```python
from build123d import *

# Parameters (mm, degrees)
SKETCH1_R                 = 25
BOSS_EXTRUDE1_DEPTH       = 10
FILLET1_R                 = 1
SKETCH2_R                 = 8
BOSS_EXTRUDE2_DEPTH       = 63.5
M8X1_0_TAPPED_HOLE1_D     = 7
M8X1_0_TAPPED_HOLE1_DEPTH = 12
M8X1_0_TAPPED_HOLE1_TIP   = 2.103012167
SKETCH5_OUTSIDE_W         = 72.398
SKETCH5_OUTSIDE_H         = 72.398
SKETCH5_OUTSIDE_W_2       = 13
SKETCH5_OUTSIDE_H_2       = 18.1448046
CUT_EXTRUDE1_DEPTH        = 5


with BuildPart() as part:
    # Sketch1 → Boss-Extrude1 (new body)
    with BuildSketch(Plane(origin=(0, 0, 0), x_dir=(1, 0, 0), z_dir=(0, 1, 0))):
        with Locations(Location((0, 0, 0), (0, 0, 270))):
            Circle(SKETCH1_R)
    extrude(amount=BOSS_EXTRUDE1_DEPTH)

    # Fillet1
    fillet1_edges = [part.edges().sort_by_distance(p)[0] for p in [
        (0, 0, -25),
        (0, 10, -25),
    ]]
    fillet(fillet1_edges, radius=FILLET1_R)

    # Sketch2 → Boss-Extrude2 (add)
    with BuildSketch(Plane(origin=(0, 10, 0), x_dir=(1, 0, 0), z_dir=(0, 1, 0))):
        with Locations(Location((0, 0, 0), (0, 0, 270))):
            Circle(SKETCH2_R)
    extrude(amount=BOSS_EXTRUDE2_DEPTH)

    # M8x1.0 Tapped Hole1
    with Locations(Plane(origin=(0, 73.5, 0), x_dir=(1, 0, 0), z_dir=(0, 1, 0))):
        with Locations((0, 0)):
            Hole(M8X1_0_TAPPED_HOLE1_D / 2, depth=M8X1_0_TAPPED_HOLE1_DEPTH)
            with Locations((0, 0, -(M8X1_0_TAPPED_HOLE1_DEPTH + M8X1_0_TAPPED_HOLE1_TIP / 2))):  # 118° drill point
                Cone(0, M8X1_0_TAPPED_HOLE1_D / 2, M8X1_0_TAPPED_HOLE1_TIP, mode=Mode.SUBTRACT)

    # Sketch5 outside → Cut-Extrude1 (cut)
    with BuildSketch(Plane(origin=(0, 73.5, 0), x_dir=(1, 0, 0), z_dir=(0, 1, 0))):
        Rectangle(SKETCH5_OUTSIDE_W, SKETCH5_OUTSIDE_H)
        Rectangle(SKETCH5_OUTSIDE_W_2, SKETCH5_OUTSIDE_H_2, mode=Mode.SUBTRACT)
    extrude(amount=-CUT_EXTRUDE1_DEPTH, mode=Mode.SUBTRACT)


solid = part.part
```
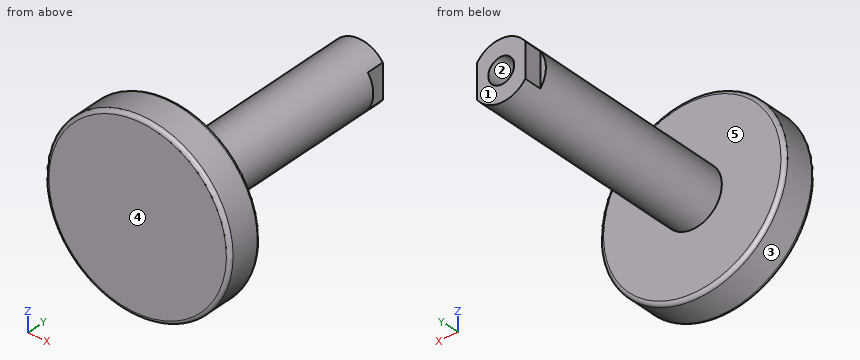
CAD build for the part. Positions are in the model's coordinates, mm. Face numbers are marked on the shaded views. A direction names the side the tool comes from. Round coordinates to 2 decimals unless told otherwise and drop trailing zeros. Order: outer loops, then holes, each group sorted by start corner. A loop starts at its lowest first (then second) coordinate and runs counter-clockwise, first axis right, second up. Notation, with made-up numbers: (55.5, 84) - (78.5, 84) arc R17 ccw to (78.5, 98) - close; hole circle Ø7 at (-34, 41). An arc over 180 degrees is marked (long way). Use CSV: the item, a comma, the result in double quotes. Start each with the question number.
1) Saw through at A-A (y = 35.5). List the corners of the cut face in (x, z), and give its area (3 significant figures).
2) Tool access for the marked faces 4 and 5: list every direction of +Z, -Z, +X, -X, +Y, -Y with a clear straight run to the whole face (end or side of a thin tool).
3) Wall check: L1, parallel to Z at x = 0, y = 65.5; L2, parallel to Y at x = -7, z = -3; L3, parallel to Y at x = 16, z = -17. Give the ranges that are in metal, low to high. Write a range as [from, to].
4) Pin check, flat tips, straight feed: pin 1 Ø10 at (x, y) = (-6.5, 11.5) entering from +Z; pin 2 Ø0.8 at (x, z) = (7.5, 0.5) entering from +Y; pin 3 Ø6 at (x, z) = (-15.5, -10) entering from +Y; pin 4 Ø6 at (x, z) = (-1, -6.5) entering from -Y. Stop position of each tip, or through.
5) Two-plate mould, pull along X, no slides. Class the marked faces 1, 2 and 3: pulls with the +X half, pulls with the -X half, needs draft (parallel to the pull), parting line crosses it, or undercut.
Values follow:
1,outline,"circle Ø16 at (0, 0)"
1,area,"201 mm2"
2,face 4,"+Z, -Z, +X, -X, -Y"
2,face 5,"+Y"
3,L1,"z = [-8, -3.5], [3.5, 8]"
3,L2,"y = [0, 68.5]"
3,L3,"y = [0, 10]"
4,pin 1,"stops at z = 24.91"
4,pin 2,"stops at y = 68.5"
4,pin 3,"stops at y = 10"
4,pin 4,"stops at y = 0"
5,face 1,"needs draft"
5,face 2,"undercut"
5,face 3,"parting line crosses it"
